Read the model definition and answer for the solid it produces. Units are mm, in the model's axes. A direction names the side the tool comes from. Coordinates: 2 decimals unless noted, no trailing zeros. Order: outer loops, then holes, each group sorted by start corner. A loop starts at its lowest first (then second) coordinate and runs counter-clockwise, first axis right, second up. Notation, with made-up numbers: M 23.25,58.25 L 45.25,58.25 A33 ccw 45.25,93.25 Z; hole C -2,-1.5 d1. An arc over 180 degrees is marked long. Use a Markdown table: item, result. Add a question column.
1) Each of these flat-tipped pins is pushed along its axis until it touches: pin 1 Ø2 at (y, z) = (-350, 32.5) entering from +X; pin 2 Ø8 at (y, z) = (-263.5, 79.5) entering from -X. Where does it stop, or does it pass through?
2) Find the intervals of material crossed by probe 1 along Y at (x, z) = (788.5, 43), in increasing order. Write a range as [from, to].
3) The mould has two halves that part along X. Classify faces 6 (the face through (922.041, -220, 50)), 7 (the face through (2572, -38.1, 63)), 8 (the face through (2579.835, -18.783, 50.089)): released by +X, released by -X, zero draft, split by the parting line, or undercut.
4) For faces 1 (the face through (51, -406.4, 29)), 2 (the face through (1287.462, -220, 50)), 3 (the face through (1290, 0, 52)), 4 (the face through (1349, -24, 101.6)), 5 (the face through (2572, -406.4, 63)), determine the directions among +Z, -Z, +X, -X, +Y, -Y from which every point of the face is accessible in a straight line to the end or side of a thin tool.
5) Find section A-A on x = 228. Write down the section's boundary in (y, z), plus the area to 3 significant figures.
6) Find section C-C on z = 36. Count the separate pieces of the cut face and the enclosed holes in it, plus the area to 3 significant figures.
7) Find section B-B on y = -140. Write down the section's boundary in (x, z).
from build123d import *

# Parameters (mm, degrees)
F1_DEPTH = 38.1
F2_W     = 38.1
F2_H     = 101.6
F3_DEPTH = 368.3
F4_W     = 38.1
F4_H     = 101.6
F5_DEPTH = 38.1


# Not quite as in the source:
# - a feature names something its author has since deleted; it is built from what else it names


with BuildPart() as f1:
    # F0 (on Front) → F1 (new body)
    with BuildSketch(Plane.XZ):
        Polygon((71.1410858821, 101.6), (0, 0), (2544.7625, 0), (2615.9035858821, 101.6), align=None)
    extrude(amount=F1_DEPTH)

    # F2 (on face) → F3 (join)
    with BuildSketch(Plane.XZ.offset(38.1)):
        with Locations((90.1910858821, 50.8)):
            Rectangle(F2_W, F2_H)
        with Locations((496.5910858821, 50.8)):
            Rectangle(F2_W, F2_H)
        with Locations((902.9910858821, 50.8)):
            Rectangle(F2_W, F2_H)
        with Locations((1306.5125, 50.8)):
            Rectangle(F2_W, F2_H)
        with Locations((1712.9125, 50.8)):
            Rectangle(F2_W, F2_H)
        with Locations((2119.3125, 50.8)):
            Rectangle(F2_W, F2_H)
        with Locations((2525.7125, 50.8)):
            Rectangle(F2_W, F2_H)
    extrude(amount=F3_DEPTH)

    # F4 (on face) → F5 (join)
    with BuildSketch(Plane.XZ.offset(406.4)):
        Polygon((2615.9035858821, 101.6), (109.2410858821, 101.6), (109.2410858821, 0), (2544.7625, 0), align=None)
        with Locations((90.1910858821, 50.8)):
            Rectangle(F4_W, F4_H)
        Polygon((71.1410858821, 101.6), (0, 0), (71.1410858821, 0), align=None)
    extrude(amount=F5_DEPTH)


solid = f1.part
Check result:
| question | item | result |
|---|---|---|
| 1 | pin 1 | stops at x = 2544.76 |
| 1 | pin 2 | stops at x = 71.14 |
| 2 | probe 1 | y = [-444.5, -406.4], [-38.1, 0] |
| 3 | face 6 | undercut |
| 3 | face 7 | zero draft |
| 3 | face 8 | released by +X |
| 4 | face 1 | +Z, -Z, -X |
| 4 | face 2 | +Z, -Z |
| 4 | face 3 | +Z, -Z, +X, -X, +Y |
| 4 | face 4 | +Z, +X, -X, +Y, -Y |
| 4 | face 5 | +Z, -Z, +X |
| 5 | outline | M -444.5,0 L -406.4,0 L -406.4,101.6 L -444.5,101.6 Z; M -38.1,0 L 0,0 L 0,101.6 L -38.1,101.6 Z |
| 5 | area | 7,740 mm2 |
| 6 | separate pieces | 1 |
| 6 | enclosed holes | 6 |
| 6 | area | 292,000 mm2 |
| 7 | outline | M 71.14,0 L 109.24,0 L 109.24,101.6 L 71.14,101.6 Z; M 477.54,0 L 515.64,0 L 515.64,101.6 L 477.54,101.6 Z; M 883.94,0 L 922.04,0 L 922.04,101.6 L 883.94,101.6 Z; M 1287.46,0 L 1325.56,0 L 1325.56,101.6 L 1287.46,101.6 Z; M 1693.86,0 L 1731.96,0 L 1731.96,101.6 L 1693.86,101.6 Z; M 2100.26,0 L 2138.36,0 L 2138.36,101.6 L 2100.26,101.6 Z; M 2506.66,0 L 2544.76,0 L 2544.76,101.6 L 2506.66,101.6 Z |
